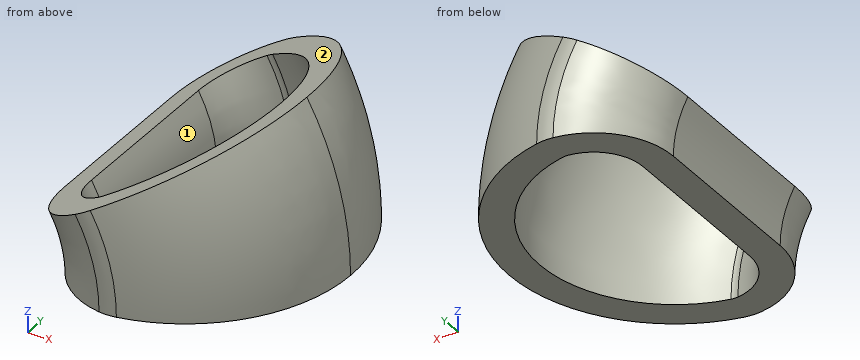
Autodesk Inventor part; units mm, degrees
ref_plane "Work Plane1" through (-7, 0, -29.5697) normal (1, 0, 0) x (0, 0, -1)
ref_plane "YZ Plane" through (0, 0, 0) normal (1, 0, 0) x (0, 1, 0)
ref_plane "XZ Plane" through (0, 0, 0) normal (0, 1, 0) x (-1, 0, 0)
sketch "Sketch1" plane through (0, 0, 0) normal (0, 0, 1) x (1, 0, 0)
  line L0 (0, 0) -> (0, 16.1) construction
  line L1 (10.73, 8.24) -> (10.73, -8.24)
  line L2 (18.59, 16.1) -> (18.59, -16.1) construction
  arc A0 (17.6161, 16.0394) -> (10.73, 8.24) centre (18.59, 8.24) ccw
  arc A1 (10.73, -8.24) -> (17.6161, -16.0394) centre (18.59, -8.24) ccw
  arc A2 (19.284, -15.9668) -> (19.284, 15.9668) centre (15.8602, 0) ccw
  line L3 (0, 0) -> (51.4073, 0)
  arc A3 (19.284, 15.9668) -> (17.6161, 16.0394) centre (18.2356, 11.078) ccw
  arc A4 (17.6161, -16.0394) -> (19.284, -15.9668) centre (18.2356, -11.078) ccw
  arc A5 (18.655, 13.0335) -> (17.9878, 13.0626) centre (18.2356, 11.078) ccw
  arc A6 (17.9878, 13.0626) -> (13.73, 8.24) centre (18.59, 8.24) ccw
  line L4 (13.73, 8.24) -> (13.73, -8.24)
  arc A7 (13.73, -8.24) -> (17.9878, -13.0626) centre (18.59, -8.24) ccw
  arc A8 (17.9878, -13.0626) -> (18.655, -13.0335) centre (18.2356, -11.078) ccw
  arc A9 (18.655, -13.0335) -> (18.655, 13.0335) centre (15.8602, 0) ccw
  point P0 (10.73, 0)
  point P1 (32.19, 0)
  point P2 (18.59, 0)
  dimension "MaxHeight" = 16.1
  dimension "FlatHeightx2" = 16.48
  dimension "ID" = 21.46
  dimension "OD" = 64.38
  dimension "d5" = 32.2
  dimension "RadAtPeak" = 18.59
  dimension "d90" = 5
  dimension "d97" = 3
revolve "Revolution1" add sketch "Sketch1" angle 30 about axis through (0, 0, 0) along (0, -1, 0) contours A0 A3 A2 L3 A9 A5 A6 L4 L1 | L3 L4 A7 A8 A9 A2 A4 A1 L1
sketch "Sketch13" plane through (10.73, -8.24, 0) normal (0, 0, -1) x (-1, 0, 0)
  arc A0 (0, 16.48) -> (-6.8861, 24.2794) centre (-7.86, 16.48) ccw
  arc A1 (-6.8861, 24.2794) -> (-8.554, 24.2068) centre (-7.5056, 19.318) ccw
  arc A2 (-8.554, 24.2068) -> (-8.6304, 24.1903) centre (-5.1302, 8.24) ccw
  arc A3 (-8.554, -7.7268) -> (-6.8861, -7.7994) centre (-7.5056, -2.838) ccw
  arc A4 (-6.8861, -7.7994) -> (0, 0) centre (-7.86, 0) ccw
  line L0 (0, 16.48) -> (0, 0)
  line L1 (-7.86, 0) -> (3, 0)
  line L2 (3, 0) -> (3, 16.48)
  line L3 (3, 16.48) -> (-7.86, 16.48)
  line L4 (-7.86, 16.48) -> (-7.86, 0)
  arc A5 (-8.6304, 24.1903) -> (-8.6304, -7.7103) centre (-5.1302, 8.24) ccw
  point P0 (10.73, 8.24)
  point P1 (-4.6967, 8.3392)
  dimension "d93" = 3
sketch "Sketch7" plane through (0, 0, 0) normal (0, 1, 0) x (-1, 0, 0)
  circle A0 centre (0, 0) radius 198.9616
sketch "Sketch8" plane through (0, 0, 0) normal (1, 0, 0) x (0, 1, 0)
  circle A0 centre (0, 0) radius 159.0195
sketch "Sketch9" plane through (0, 0, 0) normal (1, 0, 0) x (0, 0, -1)
  line L0 (74, 0) -> (35, 0)
  point P0 (0, 0)
  point P1 (-52.5, 0)
  point P2 (0, 0)
  point P3 (52.5, 0)
  dimension "d88" = 105
  dimension "d89" = 52.5
sketch "Sketch11" plane through (0, 0, 0) normal (1, 0, 0) x (0, 0, -1)
  arc A0 (-35, 25.9107) -> (-42.6927, 34.8921) centre (-44.0893, 25.9107) ccw
  line L0 (-35, 25.9107) -> (-35, 0)
  line L1 (-35, 0) -> (35, 0)
  arc A1 (-50.0415, 0) -> (-54.9585, 0) centre (-52.5, 0) ccw
  arc A2 (-50.0415, 0) -> (-54.9585, 0) centre (-37.5, 0) ccw
  arc A3 (-39.8678, 39.0634) -> (-73, 0) centre (-33.4058, 0) ccw
  arc A4 (-29.5697, 27.789) -> (-36.4391, 38.3935) centre (-44.0893, 25.9107) ccw
  line L2 (-29.5697, 27.789) -> (-29.5697, 0)
  line L3 (-35, 0) -> (35, 0)
  line L4 (-73, 0) -> (-29.5697, 0)
  arc A5 (-36.4391, 38.3935) -> (-39.8678, 39.0634) centre (-39.0518, 34.1304) ccw
  point P0 (0, 0)
  point P1 (-35, 0)
  point P2 (-29.5697, 0)
  point P3 (-54.9585, 0)
  point P4 (-50.0415, 0)
  dimension "d91" = 5
sketch "Sketch6" plane through (0.6222, 0, 0.3592) normal (-0.5, 0, 0.866) x (0, 1, 0)
  line L0 (-8.24, -10.0116) -> (8.24, -10.0116)
  arc A0 (-15.9668, -18.5655) -> (15.9668, -18.5655) centre (0, -15.1418) ccw
  arc A1 (-17.2892, -21.2298) -> (17.2892, -21.2298) centre (0, -15.1418) ccw
  line L1 (15.9668, -18.5655) -> (15.4028, -18.5655)
  arc A2 (17.2892, -21.2298) -> (15.4028, -18.5655) centre (15.4028, -20.5655) ccw
  line L2 (-15.4028, -18.5655) -> (-15.9668, -18.5655)
  arc A3 (-15.4028, -18.5655) -> (-17.2892, -21.2298) centre (-15.4028, -20.5655) ccw
  line L3 (-25.2101, 0.7184) -> (25.2101, 0.7184)
  point P0 (0, 0.7184)
  point P1 (-18.0072, -18.5655)
  point P2 (18.0072, -18.5655)
  point P3 (15.9503, -18.6419)
  point P4 (-15.9503, -18.6419)
  dimension "d47" = 2
  dimension "d48" = 2
  dimension "d49" = 2
equation "\"d5\" = 2 * MaxHeight"
equation "\"d63_Copy\" = 35"
properties part number "L_Notch1-Wedge" material "UHMW, White"
Work out the finished part from the listing and answer in its coordinate system (mm). Face numbers are marked on the shaded views. Coordinates: 2 decimals unless noted, no trailing zeros.
1. Consider line 1 along Y through (x, z) = (24.5, 9.25); line 2 along X through (y, z) = (5.5, 3.5); line 3 along Y through (x, z) = (18.5, 8). Determine where each line is inside the solid, lowest interval first.
Results list:
line 1: y = -12.65 to -8.43, 8.43 to 12.65
line 2: x = 10.14 to 13.28, 27.78 to 31.04
line 3: y = -15.75 to -12.62, 12.62 to 15.75
2. Flat-ended cylindrical pins translate along their axes: pin 1 (6 mm diameter, centred on x = 29.5, z = 6.5, fed in from +Y); pin 2 (2 mm diameter, centred on x = 21, z = 12.5, fed in from +Y); pin 3 (2 mm diameter, centred on x = 17, y = -10, fed in from -Z); pin 4 (5 mm diameter, centred on y = -10.5, z = 11.5, fed in from +X). Find the tip coordinate at first contact, or state that the pin passes through.
Results list:
pin 1: stops at y = 11.74
pin 2: stops at y = 14.44
pin 3: passes through
pin 4: stops at x = 28.09
3. For a pull along Y with two mould halves and no side action, classify the marked faces 1 and 2 as +Y half, -Y half, draft (parallel to the pull), parting line (faces both ways), or undercut.
Results list:
face 1: undercut
face 2: draft
